Can you work these out from the model? Positions are in its coordinate system, mm. A direction names the side the tool comes from. Coordinates: 2 decimals unless noted, no trailing zeros. Loops run counter-clockwise (first coordinate to the right, second up) from the corner with the lowest first, then second, coordinate; pieces in that order, holes last. Notation, with made-up numbers: (56, -7.75) -> (91, -7.75) arc R20 cw to (91, 21.25) -> close; hole circle Ø11 at (-38.5, 79). An arc over 180 degrees is marked (long way). Use one line per item in the form item = value. Start each with the question number.
(1) Imagine slicing it at C-C (y = 17). List the corners of the cut face in (x, z) for me, plus the area to 3 significant figures.
(2) Imagine slicing it at B-B (x = 0). List the corners of the cut face in (y, z) for me.
(3) I'm going to push flat-ended pins straight in: pin 1 (4.5 mm diameter, centred on x = -22, y = -8, fed in from +Z); pin 2 (1.5 mm diameter, centred on y = -23.5, z = 10.5, fed in from +X); pin 3 (1 mm diameter, centred on x = -14, z = 6.5, fed in from -Y). Where does each tip first touch, or does it pass through?
(4) Thinking about a two-plate mould opening in X: for faces 5 (the flat face through (23.55, 12.73, 4.22)), 6 (the flat face through (0, 0, 2)), 7 (the flat face through (28, 4, 6.5)), 8 (the cylindrical face through (30.5, -12.6, 1)), which applies, released by +X, released by -X, zero draft, split by the parting line, or undercut?
(5) Imagine slicing it at A-A (z = 7.5). List the corners of the cut face in (x, y) for me, plus the area to 3 significant figures.
(6) Imagine slicing it at D-D (x = 25). List the corners of the cut face in (y, z) for me.
(7) On a 3-axis mill with a long thin cutter (end or side, diameter ignored), from which of +Z, -Z, +X, -X, +Y, -Y can I reach the whole of each face in a straight line? I mean faces 1 (the flat face through (12.95, -24, 9)), 2 (the flat face through (-23.751, 12.382, 4.219)), 3 (the flat face through (-23.55, -10.73, 4.22)), 4 (the flat face through (0, -26.76, 6)). Say none if no direction works.
(8) I need wall thicknesses on line 1 (Y direction, x = -14.5, z = 14.5); line 2 (Y direction, x = -0.5, z = 4.25); line 3 (Z direction, x = 11, y = -11.5). Which ranges of each line are inside material? Lowest first, please. Write a range as [from, to].
```python
from build123d import *

# Parameters (mm, degrees)
SKETCH1_R           = 33
BOSS_EXTRUDE1_DEPTH = 2
BOSS_EXTRUDE2_DEPTH = 4.5
BOSS_EXTRUDE3_DEPTH = 10


with BuildPart() as part:
    # Sketch1 → Boss-Extrude1 (new body)
    with BuildSketch(Plane.XY):
        Circle(SKETCH1_R)
    extrude(amount=BOSS_EXTRUDE1_DEPTH)

    # Sketch3 → Boss-Extrude2 (add)
    with BuildSketch(Plane.XY.offset(2)):
        Polygon((-15.533974596, 24.61473671), (-29.745299462, 0), (-17.182050808, -21.760184977), (-12.95, -21.760184977), (-12.95, -25.760184977), (12.95, -25.760184977), (12.95, -21.760184977), (17.182050808, -21.760184977), (29.745299462, 0), (15.533974596, 24.61473671), (16.4, 25.11473671), (30.9, 0), (15.45, -26.760184977), (-15.45, -26.760184977), (-30.9, 0), (-16.4, 25.11473671), align=None)
    extrude(amount=BOSS_EXTRUDE2_DEPTH)

    # Sketch4 → Boss-Extrude3 (add)
    with BuildSketch(Plane.XY.offset(6.5)):
        Polygon((-12.95, -21.760184977), (-18.336751346, -21.760184977), (-15.45, -26.760184977), (-12.95, -26.760184977), align=None)
        Polygon((12.95, -21.760184977), (12.95, -26.760184977), (15.45, -26.760184977), (18.336751346, -21.760184977), align=None)
    extrude(amount=BOSS_EXTRUDE3_DEPTH)


solid = part.part
```
Worked out:
q1.outline = (-28.28, 0) -> (28.28, 0) -> (28.28, 2) -> (21.09, 2) -> (21.09, 6.5) -> (19.93, 6.5) -> (19.93, 2) -> (-19.93, 2) -> (-19.93, 6.5) -> (-21.09, 6.5) -> (-21.09, 2) -> (-28.28, 2) -> close
q1.area = 124 mm2
q2.outline = (-33, 0) -> (33, 0) -> (33, 2) -> (-25.76, 2) -> (-25.76, 6.5) -> (-26.76, 6.5) -> (-26.76, 2) -> (-33, 2) -> close
q3.pin_1 = 2
q3.pin_2 = 17.77
q3.pin_3 = -26.76
q4.face_5 = released by +X
q4.face_6 = undercut
q4.face_7 = zero draft
q4.face_8 = split by the parting line
q5.outline = (-18.34, -21.76) -> (-15.45, -26.76) -> (-12.95, -26.76) -> (-12.95, -21.76) -> close; (12.95, -26.76) -> (15.45, -26.76) -> (18.34, -21.76) -> (12.95, -21.76) -> close
q5.area = 39.4 mm2
q6.outline = (-21.54, 0) -> (21.54, 0) -> (21.54, 2) -> (10.22, 2) -> (10.22, 6.5) -> (8.22, 6.5) -> (8.22, 2) -> (-8.22, 2) -> (-8.22, 6.5) -> (-10.22, 6.5) -> (-10.22, 2) -> (-21.54, 2) -> close
q7.face_1 = +Z, +Y
q7.face_2 = +Z, -X, +Y
q7.face_3 = +Z
q7.face_4 = +Z, +X, -X, -Y
q8.line_1 = [-26.76, -21.76]
q8.line_2 = [-26.76, -25.76]
q8.line_3 = [0, 2]
